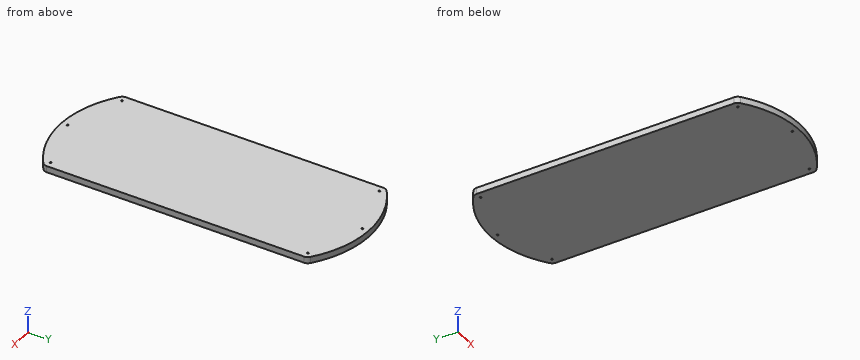
```python
from build123d import *

# Parameters (mm, degrees)
F0_R     = 1.7272
F1_DEPTH = 12.7


with BuildPart() as f1:
    # F0 (on Top) → F1 (new body)
    with BuildSketch(Plane.XY):
        with BuildLine():
            Line((127, -262.221193), (127, 262.221193))
            ThreePointArc((127, 262.221193), (125.659225, 267.900805), (121.92, 272.381193))
            ThreePointArc((121.92, 272.381193), (0, 313.021193), (-121.92, 272.381193))
            ThreePointArc((-121.92, 272.381193), (-125.659225, 267.900805), (-127, 262.221193))
            Line((-127, 262.221193), (-127, -262.221193))
            ThreePointArc((-127, -262.221193), (-125.659225, -267.900805), (-121.92, -272.381193))
            ThreePointArc((-121.92, -272.381193), (0, -313.021193), (121.92, -272.381193))
            ThreePointArc((121.92, -272.381193), (125.659225, -267.900805), (127, -262.221193))
        make_face()
        with Locations((-114.3, -262.221193)):
            Circle(F0_R, mode=Mode.SUBTRACT)
        with Locations((0, -300.321193)):
            Circle(F0_R, mode=Mode.SUBTRACT)
        with Locations((114.3, -262.221193)):
            Circle(F0_R, mode=Mode.SUBTRACT)
        with Locations((-114.3, 262.221193)):
            Circle(F0_R, mode=Mode.SUBTRACT)
        with Locations((0, 300.321193)):
            Circle(F0_R, mode=Mode.SUBTRACT)
        with Locations((114.3, 262.221193)):
            Circle(F0_R, mode=Mode.SUBTRACT)
    extrude(amount=F1_DEPTH)


solid = f1.part
```
For this review, take the finished solid that the model builds, in its own axes (mm). Coordinates: 2 decimals unless noted, no trailing zeros. Order: outer loops, then holes, each group sorted by start corner. A loop starts at its lowest first (then second) coordinate and runs counter-clockwise, first axis right, second up. Notation, with made-up numbers: (41.25, 88) -> (89.25, 88) arc R27 ccw to (89.25, 109) -> close; hole circle Ø5 at (-31, 7). An arc over 180 degrees is marked (long way). Answer as CSV lines item,"result".
Q1. We need section B-B (x = -106.5). State the section outline as (y, z) points, plus the area to 3 significant figures.
Model answer:
outline,"(-282.88, 0) -> (282.88, 0) -> (282.88, 12.7) -> (-282.88, 12.7) -> close"
area,"7,190 mm2"
Q2. Clearance check with a flat-ended pin moving along its axis: pin 1 Ø2 at (x, y) = (114.3, -262.22) entering from +Z. State where the tip first meets the part, or that it passes through.
Model answer:
pin 1,"passes through"
Q3. Wall thickness on line 1 along Y through (x, z) = (0, 6.75); line 2 along Y through (x, z) = (-114.3, 6.5); line 3 along Y through (x, z) = (-42, 3.5): over which ranges is each line inside the solid? List them lowest first. Write a range as [from, to].
Model answer:
line 1,"y = [-313.02, -302.05], [-298.59, 298.59], [302.05, 313.02]"
line 2,"y = [-277.83, -263.95], [-260.49, 260.49], [263.95, 277.83]"
line 3,"y = [-308.63, 308.63]"
Q4. We need section A-A (z = 3.5). State the section outline as (x, y) points.
Model answer:
outline,"(-127, -262.22) arc R12.7 ccw to (-121.92, -272.38) arc R203.2 ccw to (121.92, -272.38) arc R12.7 ccw to (127, -262.22) -> (127, 262.22) arc R12.7 ccw to (121.92, 272.38) arc R203.2 ccw to (-121.92, 272.38) arc R12.7 ccw to (-127, 262.22) -> close; hole circle Ø3.45 at (-114.3, -262.22); hole circle Ø3.45 at (-114.3, 262.22); hole circle Ø3.45 at (0, -300.32); hole circle Ø3.45 at (0, 300.32); hole circle Ø3.45 at (114.3, -262.22); hole circle Ø3.45 at (114.3, 262.22)"
Q5. We need section C-C (x = 76). State the section outline as (y, z) points, plus the area to 3 significant figures.
Model answer:
outline,"(-298.27, 0) -> (298.27, 0) -> (298.27, 12.7) -> (-298.27, 12.7) -> close"
area,"7,580 mm2"
